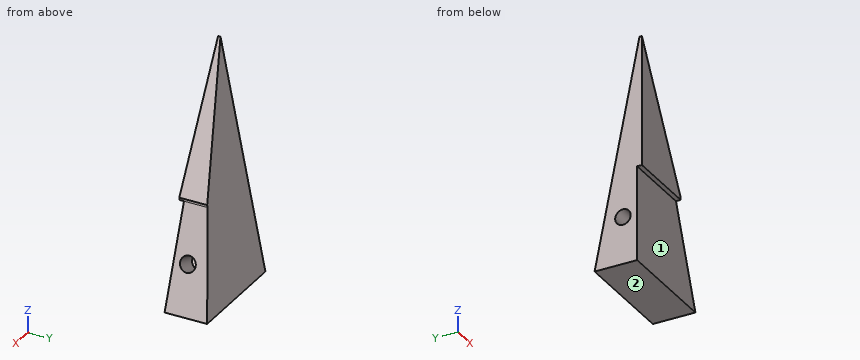
from build123d import *

# Parameters (mm, degrees)
ESBO_O1_W                                      = 130
ESBO_O1_H                                      = 20
RESSALTO_EXTRUS_O1_DEPTH                       = 95
CORTE_EXTRUS_O2_REACH                          = 22
CORTE_EXTRUS_O4_DEPTH                          = 1
CORTE_EXTRUS_O4_DEPTH_BACK                     = 46
BROCA_DE_ROSQUEAR_DE_CANO_PARA_TARRAXA_D_D     = 6.579997
BROCA_DE_ROSQUEAR_DE_CANO_PARA_TARRAXA_D_DEPTH = 10
BROCA_DE_ROSQUEAR_DE_CANO_PARA_TARRAXA_D_TIP   = 1.976830535
BROCA_DE_ROSQUEAR_DE_CANO_PARA_TARRA_2_D       = 6.579997
BROCA_DE_ROSQUEAR_DE_CANO_PARA_TARRA_2_DEPTH   = 10
BROCA_DE_ROSQUEAR_DE_CANO_PARA_TARRA_2_TIP     = 1.976830535
ESBO_O42_W                                     = 45
ESBO_O42_H                                     = 2
CORTE_EXTRUS_O5_DEPTH                          = 40


with BuildPart() as part:
    # Esboço1 → Ressalto-extrusão1 (new body)
    with BuildSketch(Plane.XY):
        Rectangle(ESBO_O1_W, ESBO_O1_H)
    extrude(amount=RESSALTO_EXTRUS_O1_DEPTH)

    # Esboço2 → Corte-extrusão2 (cut, up to next)
    with BuildSketch(Plane(origin=(0, 10, 0), x_dir=(1, 0, 0), z_dir=(0, 1, 0)), mode=Mode.PRIVATE) as corte_extrus_o2_sk1:
        Polygon((65, 0), (-20, 0), (-35, -40), (-35, -41), (-65, -95), (65, -95), align=None)
    corte_extrus_o2_tool1 = extrude(corte_extrus_o2_sk1.sketch, amount=-CORTE_EXTRUS_O2_REACH, mode=Mode.PRIVATE) & part.part
    add(corte_extrus_o2_tool1.solids().sort_by_distance((11.493506, 10, 50.911089))[0], mode=Mode.SUBTRACT)

    # Esboço13 → Corte-extrusão4 (cut, two sides)
    with BuildSketch(Plane.ZY.offset(65)) as corte_extrus_o4_sk:
        Polygon((-200.200134404, 50.040026881), (0, 10), (95, -9), (295.200134404, -49.040026881), (375.280188165, 351.360241926), (-120.120080642, 450.440295688), align=None)
    extrude(amount=CORTE_EXTRUS_O4_DEPTH, mode=Mode.SUBTRACT)
    extrude(corte_extrus_o4_sk.sketch, amount=-CORTE_EXTRUS_O4_DEPTH_BACK, mode=Mode.SUBTRACT)

    # Broca de rosquear de cano para tarraxa d
    with Locations(Plane.ZY.offset(65)):
        with Locations((20, -2)):
            Hole(BROCA_DE_ROSQUEAR_DE_CANO_PARA_TARRAXA_D_D / 2, depth=BROCA_DE_ROSQUEAR_DE_CANO_PARA_TARRAXA_D_DEPTH)
            with Locations((0, 0, -(BROCA_DE_ROSQUEAR_DE_CANO_PARA_TARRAXA_D_DEPTH + BROCA_DE_ROSQUEAR_DE_CANO_PARA_TARRAXA_D_TIP / 2))):  # 118° drill point
                Cone(0, BROCA_DE_ROSQUEAR_DE_CANO_PARA_TARRAXA_D_D / 2, BROCA_DE_ROSQUEAR_DE_CANO_PARA_TARRAXA_D_TIP, mode=Mode.SUBTRACT)

    # Broca de rosquear de cano para tarra 2
    with Locations(Plane(origin=(-17.534246575, 0, -6.575342466), x_dir=(0.351123442, 0, -0.936329178), z_dir=(0.936329178, 0, 0.351123442))):
        with Locations((-27.022468832, -2)):
            Hole(BROCA_DE_ROSQUEAR_DE_CANO_PARA_TARRA_2_D / 2, depth=BROCA_DE_ROSQUEAR_DE_CANO_PARA_TARRA_2_DEPTH)
            with Locations((0, 0, -(BROCA_DE_ROSQUEAR_DE_CANO_PARA_TARRA_2_DEPTH + BROCA_DE_ROSQUEAR_DE_CANO_PARA_TARRA_2_TIP / 2))):  # 118° drill point
                Cone(0, BROCA_DE_ROSQUEAR_DE_CANO_PARA_TARRA_2_D / 2, BROCA_DE_ROSQUEAR_DE_CANO_PARA_TARRA_2_TIP, mode=Mode.SUBTRACT)

    # Esboço42 → Corte-extrusão5 (cut)
    with BuildSketch(Plane(origin=(0, 0, 0), x_dir=(-1, 0, 0), z_dir=(0, 0, -1))):
        with Locations((42.5, -9)):
            Rectangle(ESBO_O42_W, ESBO_O42_H)
    extrude(amount=-CORTE_EXTRUS_O5_DEPTH, mode=Mode.SUBTRACT)


solid = part.part
Model file for the job. Use its own axes, mm. Face numbers are marked on the shaded views. A direction names the side the tool comes from. Round coordinates to 2 decimals unless told otherwise and drop trailing zeros. Loops run counter-clockwise (first coordinate to the right, second up) from the corner with the lowest first, then second, coordinate; pieces in that order, holes last. Notation, with made-up numbers: (14.25, 35) - (22.25, 35) arc R5 cw to (22.25, 41) - close; hole circle Ø1 at (-1, 80). An arc over 180 degrees is marked (long way). Write each question's results on one line, items separated by ' | '.
(1) Wall check: L1, parallel to Y at x = -57.5, z = 20; L2, parallel to X at y = -6, z = 36; L3, parallel to Y at x = -37, z = 6. Give the ranges that are in metal, low to high.
Answer below:
L1: y = -8 to -5.29, 1.29 to 6 | L2: x = -65 to -33.5 | L3: y = -8 to 8.8
(2) Pin check, flat tips, straight feed: pin 1 (3 mm diameter, centred on x = -52, z = 19.5, fed in from -Y); pin 2 (3 mm diameter, centred on x = -53, y = -3.5, fed in from -Z); pin 3 (10 mm diameter, centred on x = -44, z = 40, fed in from +Y); pin 4 (5.5 mm diameter, centred on y = -2, z = 20, fed in from -X). Stop position of each tip, or through.
Answer below:
pin 1: stops at y = -8 | pin 2: stops at z = 0 | pin 3: stops at y = 3 | pin 4: stops at x = -54.68
(3) 3-axis set-ups, long thin cutter, end or side, ignore diameter. For the marked faces 1 and 2: which of +Z, -Z, +X, -X, +Y, -Y reach the whole face in a straight line?
Answer below:
face 1: -Z, +X, -X, -Y | face 2: -Z, +X, -X, +Y, -Y
(4) Saw through at C-C, the plane y = 7.75. List the corners of the cut face in (x, z), then the cut area to 3 significant figures.
Answer below:
outline: (-65, 0) - (-20, 0) - (-24.22, 11.25) - (-65, 11.25) - close | area: 483 mm^2
(5) Saw through at B-B, the plane z = 57. List the corners of the cut face in (x, y).
Answer below:
outline: (-65, -10) - (-43.89, -10) - (-43.89, -1.4) - (-65, -1.4) - close
(6) Saw through at A-A, the plane x = -56. List the corners of the cut face in (y, z).
Answer below:
outline: (-10, 40) - (-8, 40) - (-8, 0) - (10, 0) - (-5.76, 78.8) - (-10, 78.8) - close; hole circle Ø6.58 at (-2, 20)
